Read the model definition and answer for the solid it produces. Units are mm, in the model's axes. Face numbers are marked on the shaded views. Coordinates: 2 decimals unless noted, no trailing zeros. Write each loop counter-clockwise with the first axis right and the second up, starting at its lowest first coordinate (ties: lowest second). Pieces come first, ordered by that corner, then holes. Notation, with made-up numbers: (6.5, 24) -> (43.5, 24) arc R11 cw to (43.5, 36) -> close; hole circle Ø5 at (63, -1). An arc over 180 degrees is marked (long way). Answer in a Markdown table with one row per item. Add a question column.
Item 1: Given pin 1 Ø2 at (x, z) = (24.5, -0.5) entering from +Y; pin 2 Ø2 at (x, z) = (2, 19) entering from +Y; pin 3 Ø0.9 at (y, z) = (1, -13.5) entering from -X, each flat-ended and moving along its own axis, determine where each tip first touches the part or whether it passes through.
Item 2: Straight lines are drawn through the part: line 1 (Z direction, x = -30, y = -0.3); line 2 (X direction, y = -0.4, z = -20); line 3 (Z direction, x = -2.5, y = 1). For each, find the intervals that lie inside material, in ascending order. Write a range as from..to.
Item 3: Section C-C on x = 30 is taken. Write down the section's boundary in (y, z).
Item 4: Section A-A on x = 0 is taken. Write down the section's boundary in (y, z).
Item 5: For a pull along Z with two mould halves and no side action, classify the marked faces 1 and 2 as +Z half, -Z half, draft (parallel to the pull), parting line (faces both ways), or undercut.
Item 6: Section D-D on y = -2.75 is taken. Write down the section's boundary in (x, z).
Item 7: Section B-B on z = 0 is taken. Write down the section's boundary in (x, y), then the cut area to 3 significant figures.
```python
from build123d import *

# Parameters (mm, degrees)
SKETCH1_W                = 65
SKETCH1_H                = 45
SKETCH1_R                = 3.9620477
SKETCH1_R_2              = 1.1
SKETCH1_W_2              = 15.2
SKETCH1_H_2              = 4
BOSS_EXTRUDE1_DEPTH      = 1.57
SKETCH1_4_W              = 15.2
SKETCH1_4_H              = 4
BOSS_EXTRUDE2_DEPTH      = 3.5
SKETCH1_5_R              = 3.9620477
BOSS_EXTRUDE3_DEPTH      = 4.5
BOSS_EXTRUDE3_DEPTH_BACK = 3.97
SKETCH2_W                = 7.81
SKETCH2_H                = 8.94
BOSS_EXTRUDE4_DEPTH      = 3.16
FILLET1_R                = 2


with BuildPart() as part:
    # Sketch1 → Boss-Extrude1 (new body)
    with BuildSketch(Plane(origin=(0, 0, 0), x_dir=(1, 0, 0), z_dir=(0, 1, 0))):
        Rectangle(SKETCH1_W, SKETCH1_H)
        Circle(SKETCH1_R, mode=Mode.SUBTRACT)
        with Locations((30, -20)):
            Circle(SKETCH1_R_2, mode=Mode.SUBTRACT)
        with Locations((30, 20)):
            Circle(SKETCH1_R_2, mode=Mode.SUBTRACT)
        with Locations((-30, 20)):
            Circle(SKETCH1_R_2, mode=Mode.SUBTRACT)
        with Locations((-30, -20)):
            Circle(SKETCH1_R_2, mode=Mode.SUBTRACT)
        with Locations((-2, -18)):
            Rectangle(SKETCH1_W_2, SKETCH1_H_2, mode=Mode.SUBTRACT)
        with Locations((19.5, -18)):
            Rectangle(SKETCH1_W_2, SKETCH1_H_2, mode=Mode.SUBTRACT)
        with Locations((-6, 18)):
            Rectangle(SKETCH1_W_2, SKETCH1_H_2, mode=Mode.SUBTRACT)
        with Locations((19.5, 18)):
            Rectangle(SKETCH1_W_2, SKETCH1_H_2, mode=Mode.SUBTRACT)
        with Locations((-2, -18)):
            Rectangle(SKETCH1_W_2, SKETCH1_H_2)
        with Locations((19.5, -18)):
            Rectangle(SKETCH1_W_2, SKETCH1_H_2)
        with Locations((-6, 18)):
            Rectangle(SKETCH1_W_2, SKETCH1_H_2)
        Circle(SKETCH1_R)
        with Locations((19.5, 18)):
            Rectangle(SKETCH1_W_2, SKETCH1_H_2)
    extrude(amount=-BOSS_EXTRUDE1_DEPTH)

    # Sketch1_4 → Boss-Extrude2 (add)
    with BuildSketch(Plane(origin=(0, 0, 0), x_dir=(1, 0, 0), z_dir=(0, 1, 0))):
        with Locations((-2, -18)):
            Rectangle(SKETCH1_4_W, SKETCH1_4_H)
        with Locations((-6, 18)):
            Rectangle(SKETCH1_4_W, SKETCH1_4_H)
        with Locations((19.5, 18)):
            Rectangle(SKETCH1_4_W, SKETCH1_4_H)
        with Locations((19.5, -18)):
            Rectangle(SKETCH1_4_W, SKETCH1_4_H)
    extrude(amount=BOSS_EXTRUDE2_DEPTH)

    # Sketch1_5 → Boss-Extrude3 (add, two sides)
    with BuildSketch(Plane(origin=(0, 0, 0), x_dir=(1, 0, 0), z_dir=(0, 1, 0))) as boss_extrude3_sk:
        Circle(SKETCH1_5_R)
    extrude(amount=BOSS_EXTRUDE3_DEPTH)
    extrude(boss_extrude3_sk.sketch, amount=-BOSS_EXTRUDE3_DEPTH_BACK)

    # Sketch2 → Boss-Extrude4 (add)
    with BuildSketch(Plane(origin=(0, 0, 0), x_dir=(1, 0, 0), z_dir=(0, 1, 0))):
        with Locations((-28.095, 12.70000129)):
            Rectangle(SKETCH2_W, SKETCH2_H)
    extrude(amount=BOSS_EXTRUDE4_DEPTH)

    # Fillet1
    fillet1_edges = [part.edges().sort_by_distance(p)[0] for p in [
        (-28.095, 3.16, -8.23000129),
        (-28.095, 3.16, -17.17000129),
    ]]
    fillet(fillet1_edges, radius=FILLET1_R)


solid = part.part
```
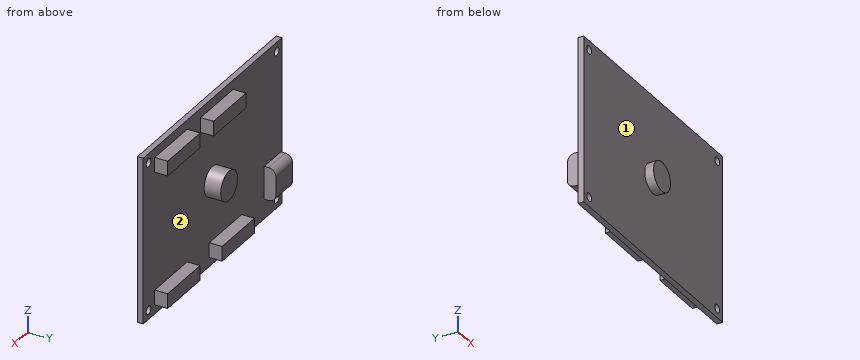
Results below:
| question | item | result |
|---|---|---|
| 1 | pin 1 | stops at y = 0 |
| 1 | pin 2 | stops at y = 3.5 |
| 1 | pin 3 | stops at x = -32 |
| 2 | line 1 | z = -22.5..-21.1, -18.9..18.9, 21.1..22.5 |
| 2 | line 2 | x = -32.5..-31.1, -28.9..28.9, 31.1..32.5 |
| 2 | line 3 | z = -20..-16, -3.07..3.07, 16..20 |
| 3 | outline | (-1.57, -22.5) -> (0, -22.5) -> (0, -21.1) -> (-1.57, -21.1) -> close; (-1.57, -18.9) -> (0, -18.9) -> (0, 18.9) -> (-1.57, 18.9) -> close; (-1.57, 21.1) -> (0, 21.1) -> (0, 22.5) -> (-1.57, 22.5) -> close |
| 4 | outline | (-3.97, -3.96) -> (-1.57, -3.96) -> (-1.57, -22.5) -> (0, -22.5) -> (0, -20) -> (3.5, -20) -> (3.5, -16) -> (0, -16) -> (0, -3.96) -> (4.5, -3.96) -> (4.5, 3.96) -> (0, 3.96) -> (0, 16) -> (3.5, 16) -> (3.5, 20) -> (0, 20) -> (0, 22.5) -> (-1.57, 22.5) -> (-1.57, 3.96) -> (-3.97, 3.96) -> close |
| 5 | face 1 | draft |
| 5 | face 2 | undercut |
| 6 | outline | circle Ø7.92 at (0, 0) |
| 7 | outline | (-32.5, -1.57) -> (-3.96, -1.57) -> (-3.96, -3.97) -> (3.96, -3.97) -> (3.96, -1.57) -> (32.5, -1.57) -> (32.5, 0) -> (3.96, 0) -> (3.96, 4.5) -> (-3.96, 4.5) -> (-3.96, 0) -> (-32.5, 0) -> close |
| 7 | area | 157 mm2 |
